Autodesk Inventor part; units mm, degrees
ref_plane "Work Plane1" through (0, 7.5, 0) normal (0, -1, 0) x (1, 0, 0)
ref_plane "YZ Plane" through (0, 0, 0) normal (1, 0, 0) x (0, 1, 0)
ref_plane "XZ Plane" through (0, 0, 0) normal (0, 1, 0) x (-1, 0, 0)
sketch "Sketch1" plane through (0, 0, 0) normal (0, 1, 0) x (-1, 0, 0)
  circle A0 centre (0, 0) radius 13
  circle A1 centre (0, 0) radius 11.5
  dimension "d0" = 26
  dimension "d1" = 23
extrude "Extrusion1" add sketch "Sketch1" along normal blind 15
sketch "Sketch2" plane through (0, 15, 0) normal (0, 1, 0) x (1, 0, 0)
  circle A0 centre (0, 0) radius 15
  circle A1 centre (0, 0) radius 11.5
  dimension "d4" = 30
extrude "Extrusion2" add sketch "Sketch2" along normal blind 2
ref_plane "Work Plane1" through (0, 7.5, 0) normal (0, -1, 0) x (1, 0, 0)
mirror "Mirror1" about plane through (0, 7.5, 0) normal (0, -1, 0) of "Extrusion2"
properties part number "inner tube"
Could you check a few things on this model? Use its own coordinates, in mm. A direction names the side the tool comes from. Give positions to 0.01 mm unless a question says otherwise; leave off trailing zeros. Loops run counter-clockwise (first coordinate to the right, second up) from the corner with the lowest first, then second, coordinate; pieces in that order, holes last. Notation, with made-up numbers: (21.25, -15.75) - (80.25, -15.75) arc R20 ccw to (80.25, -1.75) - close; hole circle Ø2 at (-2.5, -6.5). An arc over 180 degrees is marked (long way). Answer in a Markdown table with one row per item. Add a question column.
Q1. We'd pull the mould along Y, two halves only. Please class faces 3 (the face through (-8, -2, 9)), 4 (the face through (10.316, 7.395, 7.91)), 5 (the face through (-14.985, -0.986, -0.66)): +Y half, -Y half, draft (parallel to the pull), parting line (faces both ways), or undercut.
Q2. If we section it at C-C (y = 2.75): List the corners of the cut face in (x, z) for me.
Q3. Which directions (+Z, -Z, +X, -X, +Y, -Y) give clear straight access to the entire face, cutting with the end or side of a thin tool? Please do faces 1 (the face through (-0.1, 15, -13.4)), 2 (the face through (-14.985, 15.986, 0.66)).
Q4. For pin 1 (10 mm diameter, centred on x = 3.5, z = -8.5, fed in from -Y); pin 2 (5 mm diameter, centred on y = 5.5, z = 3.5, fed in from -X); pin 3 (1 mm diameter, centred on x = 10.5, z = -0.5, fed in from -Y), each with a flat end and sliding along its axis, tell me the tip position at first contact or that it passes through.
Q5. Please list where these lines run through material, in increasing order: L1, parallel to Y at x = 8, z = -11; L2, parallel to X at y = -1, z = 0; L3, parallel to X at y = 12.75, z = 1.5. Write a range as from..to.
Q6. If we section it at A-A (z = -6.25): List the corners of the cut face in (x, y) for me.
The answers:
| question | item | result |
|---|---|---|
| 1 | face 3 | -Y half |
| 1 | face 4 | undercut |
| 1 | face 5 | draft |
| 2 | outline | circle Ø26 at (0, 0); hole circle Ø23 at (0, 0) |
| 3 | face 1 | none |
| 3 | face 2 | +Y, -Y |
| 4 | pin 1 | stops at y = -2 |
| 4 | pin 2 | stops at x = -12.96 |
| 4 | pin 3 | passes through |
| 5 | L1 | y = -2..0, 15..17 |
| 5 | L2 | x = -15..-11.5, 11.5..15 |
| 5 | L3 | x = -12.91..-11.4, 11.4..12.91 |
| 6 | outline | (-13.64, -2) - (-9.65, -2) - (-9.65, 17) - (-13.64, 17) - (-13.64, 15) - (-11.4, 15) - (-11.4, 0) - (-13.64, 0) - close; (9.65, -2) - (13.64, -2) - (13.64, 0) - (11.4, 0) - (11.4, 15) - (13.64, 15) - (13.64, 17) - (9.65, 17) - close |
